Check sheet for the modelled part. Datum: model origin and axes. Units: mm. A direction names the side the tool comes from. Coordinates: 2 decimals unless noted, no trailing zeros. Loops run counter-clockwise (first coordinate to the right, second up) from the corner with the lowest first, then second, coordinate; pieces in that order, holes last. Notation, with made-up numbers: M -3,80.25 L 7,80.25 A13 cw 7,103.25 Z; hole C 88,-15.5 d10. An arc over 180 degrees is marked long. Return JSON: item names as keys, results as strings.
from build123d import *

# Parameters (mm, degrees)
F0_W     = 107.8475788236
F0_H     = 37.0553210378
F0_W_2   = 2.7404779285
F0_H_2   = 23.5804965256
F1_DEPTH = 25.4


with BuildPart() as f1:
    # F0 (on Top) → F1 (new body)
    with BuildSketch(Plane.XY):
        Rectangle(F0_W, F0_H)
        Polygon((-15.1394193599, -10.96911286), (-17.9779558206, -10.96911286), (-20.9145508137, -3.4702156283), (-30.3642967402, -3.4702156283), (-33.2647649056, -10.96911286), (-36.0413696617, -10.96911286), (-26.7206481197, 12.7094421979), (-24.4136921234, 12.7094421979), align=None, mode=Mode.SUBTRACT)
        with BuildLine():
            Line((-4.2342783753, -1.163259632), (-9.1578488908, -1.163259632))
            Line((-9.1578488908, -1.163259632), (-9.1578488908, -10.96911286))
            Line((-9.1578488908, -10.96911286), (-11.8983268193, -10.96911286))
            Line((-11.8983268193, -10.96911286), (-11.8983268193, 12.6113836656))
            Line((-11.8983268193, 12.6113836656), (-5.4316246642, 12.6113836656))
            add(Edge.make_bspline(
                [(-5.4316246642, 12.6113836656), (-1.091244367, 12.6113836656), (0.9808872494, 10.9495495922)],
                knots=[0, 0, 0, 1, 1, 1], degree=2))
            add(Edge.make_bspline(
                [(0.9808872494, 10.9495495922), (3.0530188657, 9.2877155188), (3.0530188657, 5.9485644459)],
                knots=[0, 0, 0, 1, 1, 1], degree=2))
            add(Edge.make_bspline(
                [(3.0530188657, 5.9485644459), (3.0530188657, 1.2727207488), (-1.6899175114, -0.3736303984)],
                knots=[0, 0, 0, 1, 1, 1], degree=2))
            Line((-1.6899175114, -0.3736303984), (4.7148529391, -10.96911286))
            Line((4.7148529391, -10.96911286), (1.4737603985, -10.96911286))
            Line((1.4737603985, -10.96911286), (-4.2342783753, -1.163259632))
        make_face(mode=Mode.SUBTRACT)
        Polygon((26.1793495576, -10.96911286), (23.3408130969, -10.96911286), (20.4042181039, -3.4702156283), (10.9544721773, -3.4702156283), (8.054004012, -10.96911286), (5.2773992558, -10.96911286), (14.5981207978, 12.7094421979), (16.9050767941, 12.7094421979), align=None, mode=Mode.SUBTRACT)
        with Locations((30.7906810625, 0.8211354028)):
            Rectangle(F0_W_2, F0_H_2, mode=Mode.SUBTRACT)
    extrude(amount=F1_DEPTH)


solid = f1.part
1) Section check A-A on x = -35. Record the cut outline in (y, z).
Answers:
{"outline": "M -18.53,0 L -10.97,0 L -10.97,25.4 L -18.53,25.4 Z; M -8.32,0 L 18.53,0 L 18.53,25.4 L -8.32,25.4 Z"}
2) Section check D-D on x = 22. Record the cut outline in (y, z).
Answers:
{"outline": "M -18.53,0 L -7.55,0 L -7.55,25.4 L -18.53,25.4 Z; M -0.3,0 L 18.53,0 L 18.53,25.4 L -0.3,25.4 Z"}
3) Scan lines: line 1 along Y through (x, z) = (-6.5, 21); line 2 along Y through (x, z) = (-11.5, 14.75); line 3 along X through (y, z) = (1.5, 18). Record each from-to range of solid material in increasing order. Write a range as [from, to].
Answers:
{"line 1": "[-18.53, -1.16], [12.61, 18.53]", "line 2": "[-18.53, -10.97], [12.61, 18.53]", "line 3": "[-53.92, -31.13], [-20.02, -11.9], [1.42, 10.19], [21.3, 29.42], [32.16, 53.92]"}
4) Set-up check for faces 5 (the face through (-1, -8, 25.4)), 6 (the face through (7, -10.969, 13)): record each of +Z, -Z, +X, -X, +Y, -Y from which the full face is reachable in a straight line by a thin tool's end or side.
Answers:
{"face 5": "+Z, +X, -X, +Y, -Y", "face 6": "+Z, -Z"}
5) Draft check along X on faces 1 (the face through (-9.158, -6, 13)), 2 (the face through (31, -10.969, 13)), 3 (the face through (-53.924, 0, 13)), 4 (the face through (-1, -8, 0)). Enter one of: +X half, -X half, draft (parallel to the pull), parting line (faces both ways), or undercut.
Answers:
{"face 1": "undercut", "face 2": "undercut", "face 3": "-X half", "face 4": "draft"}
6) Section check B-B on z = 21.25. Count the separate pieces of the cut face and the enclosed holes in it, then the cut area to 3 significant figures.
Answers:
{"separate pieces": "1", "enclosed holes": "4", "area": "3,320 mm²"}
7) Go/stop test with a flat-tipped pin: pin 1 Ø5 at (x, y) = (-33.5, -4) entering from -Z. Record where the tip stops, or that it passes through.
Answers:
{"pin 1": "z = 0"}
